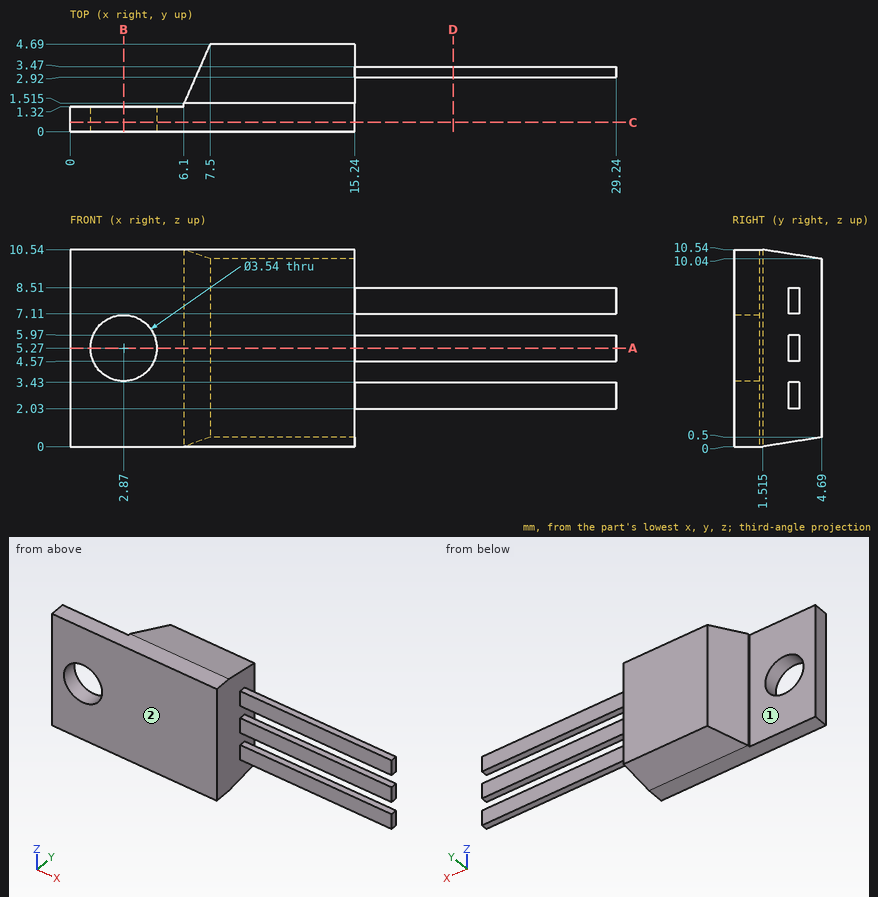
Input: dimensioned drawing with shaded views. Units: mm. Origin: part minimum x, y, z. A direction names the side the tool comes from. Round coordinates to 2 decimals unless told otherwise and drop trailing zeros. Order: outer loops, then holes, each group sorted by start corner. A loop starts at its lowest first (then second) coordinate and runs counter-clockwise, first axis right, second up. Notation, with made-up numbers: (77, 6.5) -> (96, 6.5) arc R23 ccw to (96, 23.5) -> close; hole circle Ø2 at (-18.75, 4.5). An arc over 180 degrees is marked (long way). Put each result on its own line as item: value. Start each with the question number.
Q1. Section D-D on x = 20.5. Return the cut outline in (y, z), and give its area (3 significant figures).
Q2. Line query: probe 1 along Z at (x, y) = (2.87, 0.4); probe 2 along Y at (x, z) = (27, 3.25); probe 3 along Z at (x, y) = (3.5, 1.1). Output: solid intervals per line, ascending.
Q3. Reachability of the marked faces 1 and 2 from +Z, -Z, +X, -X, +Y, -Y: full face, straight path, thin tool, end or side. Return the list, or none.
Q4. Section C-C on y = 0.5. Return the cut outline in (x, z).
Q5. Section A-A on z = 5.27. Return the cut outline in (x, y) (3 decimals).
Q6. Section B-B on x = 2.87. Return the cut outline in (y, z).
Q7. First-contact query: pin 1 (1.1 mm diameter, centred on x = 25, z = 7.5, fed in from -Y); pin 2 (3 mm diameter, centred on x = 2.87, z = 5.27, fed in from +Y); pin 3 (0.6 mm diameter, centred on x = 23, y = 3, fed in from +Z); pin 4 (5 mm diameter, centred on x = 3, z = 5.5, fed in from +Y). Flat tips, straight axial feed; report the tip coordinate or a pass-through.
Ans:
1. outline: (2.92, 2.03) -> (3.47, 2.03) -> (3.47, 3.43) -> (2.92, 3.43) -> close; (2.92, 4.57) -> (3.47, 4.57) -> (3.47, 5.97) -> (2.92, 5.97) -> close; (2.92, 7.11) -> (3.47, 7.11) -> (3.47, 8.51) -> (2.92, 8.51) -> close
1. area: 2.31 mm2
2. probe 1: z = 0 to 3.5, 7.04 to 10.54
2. probe 2: y = 2.92 to 3.47
2. probe 3: z = 0 to 3.62, 6.92 to 10.54
3. face 1: +Z, -Z, -X, +Y
3. face 2: +Z, -Z, +X, -X, -Y
4. outline: (0, 0) -> (15.24, 0) -> (15.24, 10.54) -> (0, 10.54) -> close; hole circle Ø3.54 at (2.87, 5.27)
5. outline: (0, 0) -> (1.1, 0) -> (1.1, 1.32) -> (0, 1.32) -> close; (4.64, 0) -> (15.24, 0) -> (15.24, 2.92) -> (29.24, 2.92) -> (29.24, 3.47) -> (15.24, 3.47) -> (15.24, 4.69) -> (7.5, 4.69) -> (6.1, 1.515) -> (6.1, 1.32) -> (4.64, 1.32) -> close
6. outline: (0, 0) -> (1.32, 0) -> (1.32, 3.5) -> (0, 3.5) -> close; (0, 7.04) -> (1.32, 7.04) -> (1.32, 10.54) -> (0, 10.54) -> close
7. pin 1: stops at y = 2.92
7. pin 2: passes through
7. pin 3: stops at z = 8.51
7. pin 4: stops at y = 1.32
